Geometry: final body of the model. Coordinates: model frame, mm. A direction names the side the tool comes from. Coordinates: 2 decimals unless noted, no trailing zeros. Loops run counter-clockwise (first coordinate to the right, second up) from the corner with the lowest first, then second, coordinate; pieces in that order, holes last. Notation, with made-up numbers: (59.5, 79.5) - (86.5, 79.5) arc R21 cw to (86.5, 108.5) - close; hole circle Ø6 at (-18.75, -30.5). An arc over 180 degrees is marked (long way). Put each result on its own line as item: value. Start each with the question number.
1) Section A-A on z = 5. Output: boundary loops of the cut face in (x, y).
2) Section D-D on z = 6. Output: boundary loops of the cut face in (x, y), and give its area (3 significant figures).
3) Reachability of faces 4 (the flat face through (2, -5, 5)), 5 (the flat face through (14.5, -1, 5)), 6 (the flat face through (12.2, -4.5, 6.45)), 7 (the flat face through (11, 3, 4)), 8 (the flat face through (12.2, -4.5, 3.55)) from +Z, -Z, +X, -X, +Y, -Y: full face, straight path, thin tool, end or side. Return the list, or none.
4) Section C-C on y = -2.75. Output: boundary loops of the cut face in (x, z), and give its area (3 significant figures).
5) Contact query for flat-ended pins moving along their axis: pin 1 Ø0.8 at (x, y) = (-0.5, -4.5) entering from +Z; pin 2 Ø4 at (x, z) = (10, 7) entering from +Y; pin 3 Ø1.1 at (x, z) = (7.5, 8) entering from -Y. Output: stop coordinate, or through.
6) Material intervals for line 1 along Z through (x, y) = (9.5, -2.5); line 2 along Y through (x, z) = (0, 2.5); line 3 along X through (y, z) = (-1.25, 4), sorted ascending. Write a range as from..to.
7) Draft query along X for faces 1 (the cylindrical face through (10.886, -0.944, 5.575)), 2 (the flat face through (1.9, -4.5, 3.55)), 3 (the cylindrical face through (4.76, 3.18, 5.07)). Return one class per face: +X half, -X half, draft (parallel to the pull), parting line (faces both ways), or undercut.
8) Section B-B on x = 0. Output: boundary loops of the cut face in (y, z).
```python
from build123d import *

# Parameters (mm, degrees)
SKETCH1_R                       = 3.5
MAIN_DEPTH                      = 10
SKETCH3_W                       = 20
SKETCH3_H                       = 2.9
MAKERBEAMRECTANGULARGUIDE_DEPTH = 1
SKETCH4_R                       = 1.5
MAKERBEAMFIXHOLE_DEPTH          = 9
FILLET1_R                       = 2


with BuildPart() as part:
    # Sketch1 → Main (new body)
    with BuildSketch(Plane.XY):
        with BuildLine():
            Line((-5.5, 0), (-5.5, -4))
            Line((-5.5, -4), (14.5, -4))
            Line((14.5, -4), (14.5, 3))
            Line((14.5, 3), (4.609772229, 3))
            ThreePointArc((4.609772229, 3), (-1.564648961, 5.272748205), (-5.5, 0))
        make_face()
        Circle(SKETCH1_R, mode=Mode.SUBTRACT)
    extrude(amount=MAIN_DEPTH)

    # Sketch3 → MakerBeamRectangularGuide (add)
    with BuildSketch(Plane(origin=(0, -4, 0), x_dir=(-1, 0, 0), z_dir=(0, -1, 0))):
        with Locations((-4.5, -5)):
            Rectangle(SKETCH3_W, SKETCH3_H)
    extrude(amount=MAKERBEAMRECTANGULARGUIDE_DEPTH)

    # Sketch4 → MakerBeamFixHole (cut, through all)
    with BuildSketch(Plane(origin=(0, 3, 0), x_dir=(1, 0, 0), z_dir=(0, 1, 0))):
        with Locations((9.5, -5)):
            Circle(SKETCH4_R)
    extrude(amount=-MAKERBEAMFIXHOLE_DEPTH, mode=Mode.SUBTRACT)

    # Fillet1
    fillet1_edges = [part.edges().sort_by_distance(p)[0] for p in [
        (4.609772229, 3, 5),
    ]]
    fillet(fillet1_edges, radius=FILLET1_R)


solid = part.part
```
Answer block:
1. outline: (-5.5, -5) - (8, -5) - (8, 3) - (5.59, 3) arc R2 cw to (4.1, 3.67) arc R5.5 ccw to (-5.5, 0) - close; (11, -5) - (14.5, -5) - (14.5, 3) - (11, 3) - close; hole circle Ø7 at (0, 0)
2. outline: (-5.5, -5) - (8.38, -5) - (8.38, 3) - (5.59, 3) arc R2 cw to (4.1, 3.67) arc R5.5 ccw to (-5.5, 0) - close; (10.62, -5) - (14.5, -5) - (14.5, 3) - (10.62, 3) - close; hole circle Ø7 at (0, 0)
2. area: 119 mm²
3. face 4: +Z, -Z, +X, -X, -Y
3. face 5: +Z, -Z, +X, +Y, -Y
3. face 6: +Z, +X, -X, -Y
3. face 7: +Z, -Z, +X, +Y
3. face 8: -Z, +X, -X, -Y
4. outline: (-5.5, 0) - (-2.17, 0) - (-2.17, 10) - (-5.5, 10) - close; (2.17, 0) - (14.5, 0) - (14.5, 10) - (2.17, 10) - close; hole circle Ø3 at (9.5, 5)
4. area: 150 mm²
5. pin 1: stops at z = 6.45
5. pin 2: stops at y = 3
5. pin 3: stops at y = -4
6. line 1: z = 0..3.5, 6.5..10
6. line 2: y = -4..-3.5, 3.5..5.5
6. line 3: x = -5.5..-3.27, 3.27..8.38, 10.62..14.5
7. face 1: undercut
7. face 2: draft
7. face 3: +X half
8. outline: (-5, 3.55) - (-4, 3.55) - (-4, 0) - (-3.5, 0) - (-3.5, 10) - (-4, 10) - (-4, 6.45) - (-5, 6.45) - close; (3.5, 0) - (5.5, 0) - (5.5, 10) - (3.5, 10) - close
